Autodesk Inventor part; units mm, degrees
ref_plane "YZ Plane" through (0, 0, 0) normal (1, 0, 0) x (0, 1, 0)
ref_plane "XZ Plane" through (0, 0, 0) normal (0, 1, 0) x (-1, 0, 0)
ref_plane "XY Plane" through (0, 0, 0) normal (0, 0, 1) x (1, 0, 0)
sketch "Szkic1" plane through (0, 0, 0) normal (0, 0, 1) x (1, 0, 0)
  circle A0 centre (0, 0) radius 30
  dimension "d0" = 60
extrude "Wyciągnięcie proste1" add sketch "Szkic1" along normal mid plane 5
sketch "Szkic3" plane through (0, 0, 2.5) normal (0, 0, 1) x (1, 0, 0)
  point P0 (0, 0)
sketch "Szkic4" plane through (0, 0, 2.5) normal (0, 0, 1) x (1, 0, 0)
  circle A0 centre (0, 0) radius 2.4
  dimension "d3" = 4.8
extrude "Wyciągnięcie proste2" cut sketch "Szkic4" against normal blind 5
sketch "Szkic7" plane through (0, 0, 2.5) normal (0, 0, 1) x (1, 0, 0)
  point P0 (0, 0)
sketch "Szkic11" plane through (0, 0, 2.5) normal (0, 0, 1) x (1, 0, 0)
  circle A0 centre (-25, 0) radius 4
  circle A1 centre (0, 0) radius 30
  circle A2 centre (-21.6506, -12.5) radius 4
  circle A3 centre (-12.5, -21.6506) radius 4
  circle A4 centre (0, -25) radius 4
  circle A5 centre (12.5, -21.6506) radius 4
  circle A6 centre (21.6506, -12.5) radius 4
  circle A7 centre (25, 0) radius 4
  circle A8 centre (21.6506, 12.5) radius 4
  circle A9 centre (12.5, 21.6506) radius 4
  circle A10 centre (0, 25) radius 4
  circle A11 centre (-12.5, 21.6506) radius 4
  circle A12 centre (-21.6506, 12.5) radius 4
  point P0 (19.3799, 15.793)
  point P1 (23.3671, 8.887)
  point P2 (24.68, -3.9872)
  point P3 (24.68, 3.9872)
  point P4 (23.3671, -8.887)
  point P5 (19.3799, -15.793)
  point P6 (8.887, -23.3671)
  point P7 (15.793, -19.3799)
  point P8 (3.9872, -24.68)
  point P9 (-3.9872, -24.68)
  point P10 (-15.793, -19.3799)
  point P11 (-8.887, -23.3671)
  point P12 (-19.3799, -15.793)
  point P13 (-23.3671, -8.887)
  point P14 (-24.68, -3.9872)
  point P15 (-24.68, 3.9872)
  point P16 (8.887, 23.3671)
  point P17 (15.793, 19.3799)
  point P18 (-3.9872, 24.68)
  point P19 (3.9872, 24.68)
  point P20 (-15.793, 19.3799)
  point P21 (-8.887, 23.3671)
  point P22 (-23.3671, 8.887)
  point P23 (-19.3799, 15.793)
  dimension "d15" = 25
  dimension "d16" = 0
  dimension "d17" = 8
  dimension "d20" = 360
extrude "Wyciągnięcie proste3" add sketch "Szkic11" against normal blind 5 contours A0 | A2 | A3 | A4 | A5 | A6 | A7 | A8 | A9 | A10 | A11 | A12
sketch "Szkic16" plane through (0, 0, 2.5) normal (0, 0, 1) x (1, 0, 0)
  arc A0 (30, 0) -> (30, 0) centre (-25, 0) ccw
  circle A1 centre (-25, 0) radius 2.5
  arc A2 (30, 0) -> (30, 0) centre (-25, 0) ccw
  point P0 (0, 0)
  dimension "d30" = 5
extrude "Wyciągnięcie proste4" cut sketch "Szkic16" against normal blind 5 contours A1
pattern_circular "Szyk kołowy1" count 12 over 360 about axis through (0, 0, 0) along (0, 0, 1) of "Wyciągnięcie proste4"
sketch "Szkic22" plane through (0, 0, 2.5) normal (0, 0, 1) x (1, 0, 0)
  line L0 (0, 0) -> (-4.3, 0)
  circle A0 centre (-4.3, 0) radius 0.5
  line L1 (-4.3, 0) -> (-6.4, 0)
  line L2 (-6.4, 0) -> (-8.5, 0)
  line L3 (-8.5, 0) -> (-10.6, 0)
  line L4 (-10.6, 0) -> (-12.7, 0)
  line L5 (-12.7, 0) -> (-14.8, 0)
  dimension "d51" = 4.3
  dimension "d52" = 1
  dimension "d53" = 2.1
  dimension "d54" = 2.1
  dimension "d55" = 2.1
  dimension "d56" = 2.1
  dimension "d57" = 2.1
hole "Otwór2" at (-14.8, 0, 2.5) at (-12.7, 0, 2.5) at (-10.6, 0, 2.5) at (-8.5, 0, 2.5) at (-6.4, 0, 2.5) at (-4.3, 0, 2.5) direction (0, 0, -1) diameter 1 depth 25 tip angle 118
pattern_circular "Szyk kołowy2" count 4 over 360 about axis through (0, 0, 0) along (0, 0, 1) of "Otwór2"
sketch "Szkic23" plane through (0, 0, 2.5) normal (0, 0, 1) x (1, 0, 0)
  circle A0 centre (0, 0) radius 3.75
  line L0 (0, 0) -> (3.75, 0) construction
  line L1 (-17, -3) -> (17, -3)
  line L2 (17, -3) -> (17, 3)
  line L3 (17, 3) -> (-17, 3)
  line L4 (-17, 3) -> (-17, -3)
  line L5 (-17, -3) -> (17, 3) construction
  line L6 (17, -3) -> (-17, 3) construction
  arc A1 (-17, 3) -> (-17, -3) centre (-17, 0) ccw
  arc A2 (17, -3) -> (17, 3) centre (17, 0) ccw
  point P0 (-2.25, -3)
  point P1 (2.25, -3)
  point P2 (2.25, 3)
  point P3 (-2.25, 3)
  dimension "d68" = 7.5
  dimension "d70" = 34
  dimension "d71" = 6
extrude "Wyciągnięcie proste8" cut sketch "Szkic23" against normal blind 1.5
sketch "Szkic24" plane through (0, 0, 2.5) normal (0, 0, 1) x (1, 0, 0)
  line L0 (-3, -17) -> (3, -17)
  line L1 (3, -17) -> (3, 17)
  line L2 (3, 17) -> (-3, 17)
  line L3 (-3, 17) -> (-3, -17)
  line L4 (-3, -17) -> (3, 17) construction
  line L5 (3, -17) -> (-3, 17) construction
  arc A0 (2.8188, 15.9732) -> (-2.8188, 15.9732) centre (0, 17) ccw
  arc A1 (-2.8188, -15.9732) -> (2.8188, -15.9732) centre (0, -17) ccw
  point P0 (0, 0)
  point P1 (3, 17)
  point P2 (-3, 17)
  point P3 (-3, -17)
  point P4 (3, -17)
  point P5 (3, -17)
  point P6 (-3, -17)
  point P7 (-3, 17)
  point P8 (3, 17)
  dimension "d74" = 6
  dimension "d75" = 34
  dimension "d76" = 6
  dimension "d77" = 6
extrude "Wyciągnięcie proste9" cut sketch "Szkic24" against normal blind 1.5
sketch "Szkic25" plane through (0, 0, 2.5) normal (0, 0, 1) x (1, 0, 0)
  line L0 (0, 0) -> (-10.6066, -10.6066)
  line L1 (0, 0) -> (15, 0) construction
  circle A0 centre (-10.6066, -10.6066) radius 2.5
  dimension "d80" = 15
  dimension "d81" = 135
  dimension "d82" = 5
extrude "Wyciągnięcie proste10" cut sketch "Szkic25" against normal blind 5
pattern_circular "Szyk kołowy3" count 4 over 360 about axis through (0, 0, 0) along (0, 0, 1) of "Wyciągnięcie proste10"
sketch "Szkic26" plane through (0, 0, 1) normal (0, 0, 1) x (1, 0, 0)
  circle A0 centre (0, 0) radius 2.4
  dimension "d88" = 4.8
extrude "Wyciągnięcie proste11" cut sketch "Szkic26" against normal blind 5
sketch "Szkic27" plane through (0, 0, 2.5) normal (0, 0, 1) x (1, 0, 0)
  point P0 (0, 0)
properties part number "Servo_przelozenie"
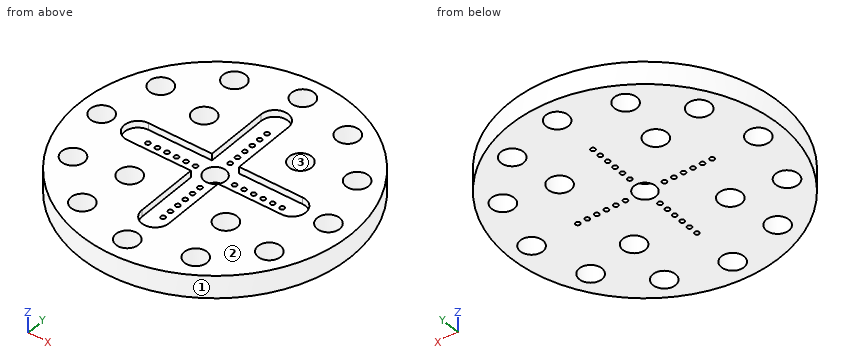
Source: CAD feature listing. Evaluate the final solid. Frame: model axes, mm. Face numbers are marked on the shaded views. Coordinates: 2 decimals unless noted, no trailing zeros. Loops run counter-clockwise (first coordinate to the right, second up) from the corner with the lowest first, then second, coordinate; pieces in that order, holes last. Notation, with made-up numbers: (50.25, 15) - (73.25, 15) arc R29 ccw to (73.25, 40) - close; hole circle Ø4 at (45, -9). An arc over 180 degrees is marked (long way). Return JSON: item names as keys, results as strings.
Q1. Contact query for flat-ended pins moving along their axis: P1, Ø6, axis at x = -21.65, y = -12.5, coming from the -Z side; P2, Ø1.6, axis at x = 9, z = 1.5, coming from the -Y side; P3, Ø1.2, axis at x = 8.5, z = 1.5, coming from the +Y side; P4, Ø1.5, axis at x = 20, z = 2, coming from the +Y side. Output: stop coordinate, or through.
Results:
{"P1": "z = -2.5", "P2": "y = -28.86", "P3": "y = 28.94", "P4": "y = 23.01"}
Q2. Section B-B, the plane x = 25. Return loops of the section in (y, z), plus the area to 3 significant figures.
Results:
{"outline": "(-16.58, -2.5) - (-2.5, -2.5) - (-2.5, 2.5) - (-16.58, 2.5) - close; (2.5, -2.5) - (16.58, -2.5) - (16.58, 2.5) - (2.5, 2.5) - close", "area": "141 mm2"}
Q3. Section A-A, the plane y = -26. Return loops of the section in (x, z), plus the area to 3 significant figures.
Results:
{"outline": "(-14.97, -2.5) - (-2.29, -2.5) - (-2.29, 2.5) - (-14.97, 2.5) - close; (2.29, -2.5) - (14.97, -2.5) - (14.97, 2.5) - (2.29, 2.5) - close", "area": "127 mm2"}
Q4. Mould query, pull axis X, two halves, no side actions, for the marked faces 1, 2 and 3. Classes: released by +X, released by -X, zero draft, split by the parting line, or undercut.
Results:
{"face 1": "split by the parting line", "face 2": "zero draft", "face 3": "undercut"}
Q5. Material intervals for line 1 along X through (y, z) = (-21.5, 1.4); line 2 along Y through (x, z) = (8.5, 1.7); line 3 along X through (y, z) = (12.5, -1.4), sorted ascending.
Results:
{"line 1": "-20.92 to -15, -10 to 10, 15 to 20.92", "line 2": "-28.77 to -11.95, -9.26 to -3, 3 to 9.26, 11.95 to 28.77", "line 3": "-27.27 to -24.15, -19.15 to -12.24, -8.97 to -0.46, 0.46 to 8.97, 12.24 to 19.15, 24.15 to 27.27"}
Q6. Section C-C, the plane z = -1.05. Give the number of separate pieces and of enclosed holes in the cut face, plus the area to 3 significant figures.
Results:
{"separate pieces": "1", "enclosed holes": "41", "area": "2,480 mm2"}
